The drawing under review shows one solid part. Ordinate dimensions are in mm from its lowest x, y, z. Give positions to 0.01 mm unless a question says otherwise; leave off trailing zeros. Order: outer loops, then holes, each group sorted by start corner. A loop starts at its lowest first (then second) coordinate and runs counter-clockwise, first axis right, second up. Notation, with made-up numbers: (68, -2.5) - (122, -2.5) arc R21 ccw to (122, 25.5) - close; hole circle Ø6 at (-33, 9). An arc over 180 degrees is marked (long way). Use CSV: the item, a comma, the result in double quotes. Start each with the question number.
1. Take a section at B-B, the plane y = 60.96. State the section outline as (x, z) points (3 decimals).
2. Take a section at C-C, the plane z = 2. State the section outline as (x, y) points (3 decimals).
3. Take a section at A-A, the plane x = 10.16. State the section outline as (y, z) points (3 decimals).
4. Draft analysis for pull direction X (two halves, no side actions). For the marked faces 1, 2, 3 and 4, state which applies: released by +X, released by -X, zero draft, split by the parting line, or undercut.
5. Take a section at D-D, the plane y = 31.5. State the section outline as (x, z) points, then the cut area to 3 significant figures.
6. For pin 1 (10 mm diameter, centred on x = 10.16, y = 60.96, fed in from +Z), flat-tipped, find the tip position at first contact; note if it passes through.
7. To check wall thickness, follow line 1 (Y direction, x = 10.16, z = 1.75) (3 decimals); line 2 (Y direction, x = 10.16, z = 11); line 3 (X direction, y = 31.5, z = 5.5). State the ranges of each line that lie inside material, in increasing order. Write a range as [from, to].
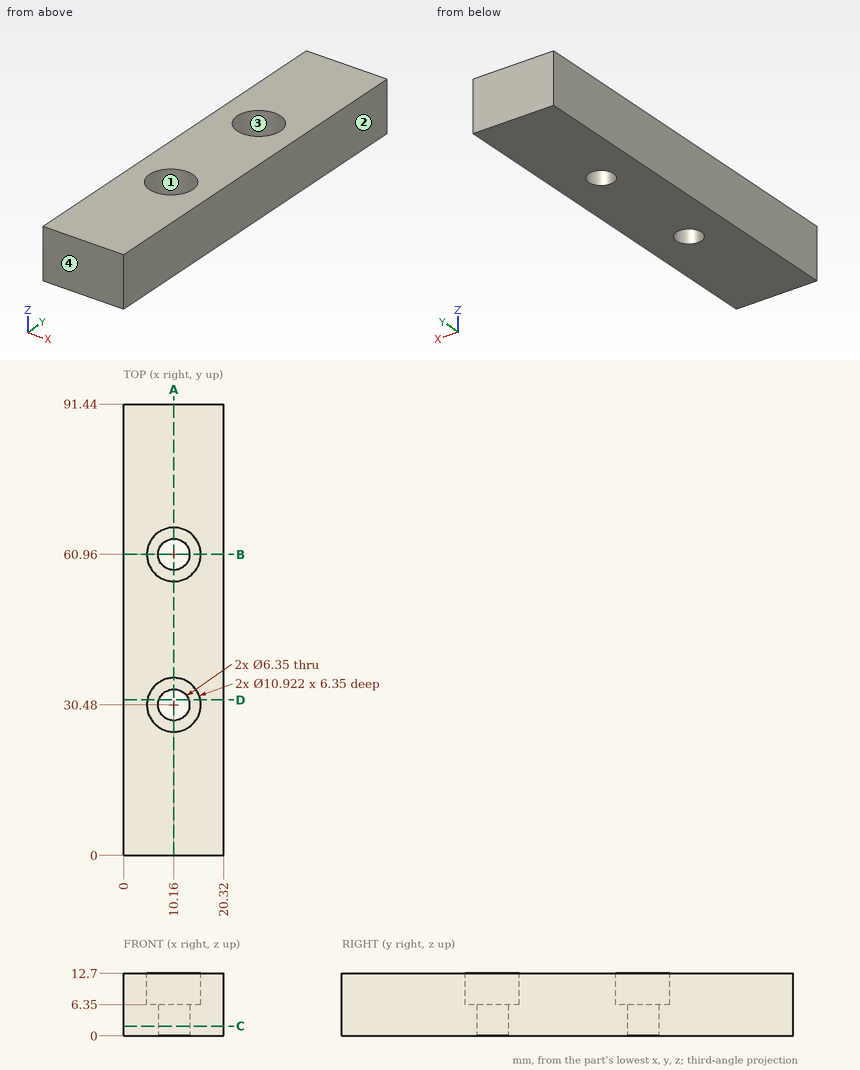
Determined:
1,outline,"(0, 0) - (6.985, 0) - (6.985, 6.35) - (4.699, 6.35) - (4.699, 12.7) - (0, 12.7) - close; (13.335, 0) - (20.32, 0) - (20.32, 12.7) - (15.621, 12.7) - (15.621, 6.35) - (13.335, 6.35) - close"
2,outline,"(0, 0) - (20.32, 0) - (20.32, 91.44) - (0, 91.44) - close; hole circle Ø6.35 at (10.16, 30.48); hole circle Ø6.35 at (10.16, 60.96)"
3,outline,"(0, 0) - (27.305, 0) - (27.305, 6.35) - (25.019, 6.35) - (25.019, 12.7) - (0, 12.7) - close; (33.655, 0) - (57.785, 0) - (57.785, 6.35) - (55.499, 6.35) - (55.499, 12.7) - (35.941, 12.7) - (35.941, 6.35) - (33.655, 6.35) - close; (64.135, 0) - (91.44, 0) - (91.44, 12.7) - (66.421, 12.7) - (66.421, 6.35) - (64.135, 6.35) - close"
4,face 1,"undercut"
4,face 2,"released by +X"
4,face 3,"undercut"
4,face 4,"zero draft"
5,outline,"(0, 0) - (7.15, 0) - (7.15, 6.35) - (4.8, 6.35) - (4.8, 12.7) - (0, 12.7) - close; (13.17, 0) - (20.32, 0) - (20.32, 12.7) - (15.52, 12.7) - (15.52, 6.35) - (13.17, 6.35) - close"
5,area,"152 mm²"
6,pin 1,"stops at z = 6.35"
7,line 1,"y = [0, 27.305], [33.655, 57.785], [64.135, 91.44]"
7,line 2,"y = [0, 25.02], [35.94, 55.5], [66.42, 91.44]"
7,line 3,"x = [0, 7.15], [13.17, 20.32]"
